from build123d import *

# Parameters (mm, degrees)
F0_W     = 274.9042
F0_H     = 560.5272
F1_DEPTH = 19.05
F3_DEPTH = 25.4
F4_W     = 50.8
F4_H     = 19.05
F5_DEPTH = 19.05
F7_DEPTH = 19.05
F8_R     = 50.8


with BuildPart() as f1:
    # F0 (on Top) → F1 (new body)
    with BuildSketch(Plane.XY):
        with Locations((-33.675123, 17.433073)):
            Rectangle(F0_W, F0_H)
    extrude(amount=F1_DEPTH)

    # F2 (on face) → F3 (cut)
    with BuildSketch(Plane.XY.offset(19.05)):
        Polygon((49.734686, 173.754715), (71.204288, 219.794873), (53.93326, 227.848758), (32.463658, 181.808599), align=None)
        Polygon((-21.578634, 65.918441), (-4.307605, 57.864557), (17.161997, 103.904715), (-0.109031, 111.958599), align=None)
        Polygon((-75.620925, -49.971717), (-58.349897, -58.025601), (-36.880294, -11.985443), (-54.151322, -3.931559), align=None)
        Polygon((-129.663216, -165.861875), (-112.392188, -173.915759), (-90.922585, -127.875601), (-108.193613, -119.821717), align=None)
    extrude(amount=-F3_DEPTH, mode=Mode.SUBTRACT)

    # F4 (on face) → F5 (join)
    with BuildSketch(Plane.XZ.offset(262.830527)):
        with Locations((-97.797423, 9.525)):
            Rectangle(F4_W, F4_H)
        with Locations((29.202577, 9.525)):
            Rectangle(F4_W, F4_H)
    extrude(amount=F5_DEPTH)

    # F6 (on face) → F7 (cut)
    with BuildSketch(Plane.XY.offset(19.05)):
        Polygon((-133.570358, -71.706755), (26.208879, 232.032016), (-133.570358, 232.032016), align=None)
    extrude(amount=-F7_DEPTH, mode=Mode.SUBTRACT)

    # F8
    f8_edges = [f1.edges().sort_by_distance(p)[0] for p in [
        (-171.127223, 297.696673, 9.525),
        (103.776977, 297.696673, 9.525),
    ]]
    fillet(f8_edges, radius=F8_R)


solid = f1.part
Model file for the job. Use its own axes, mm. A direction names the side the tool comes from. Round coordinates to 2 decimals unless told otherwise and drop trailing zeros. Loops run counter-clockwise (first coordinate to the right, second up) from the corner with the lowest first, then second, coordinate; pieces in that order, holes last.
1. Drop flat-ended pins along their axis: P1, Ø5.5, axis at y = -267.5, z = 6, coming from the -X side; P2, Ø5.5, axis at x = 75, z = 14, coming from the -Y side; P3, Ø5.5, axis at y = -267.5, z = 12, coming from the +X side. Give the stop position or say it passes through.
Check values:
P1: stops at x = -123.2
P2: stops at y = -262.83
P3: stops at x = 54.6
2. Wall check: probe 1 along Y at (x, z) = (-43, 2); probe 2 along Y at (x, z) = (-91, 9.75); probe 3 along X at (y, z) = (-6, 14.5). Give the ranges that are in metal, low to high.
Check values:
probe 1: y = -262.83 to -25.11, -9.13 to 100.47, 232.03 to 297.7
probe 2: y = -281.88 to -128.04, -127.84 to 9.22, 232.03 to 297.7
probe 3: x = -171.13 to -133.57, -99.01 to -55.12, -49.72 to 103.78
3. Mould opens along Y. For faces 1 (the flat face through (-171.127, -12, 9)), 2 (the flat face through (-119, -143, 10)), 3 (the cylindrical face through (-156.64, 282.42, 9.66)) say: +Y half, -Y half, draft (parallel to the pull), parting line (faces both ways), or undercut.
Check values:
face 1: draft
face 2: undercut
face 3: +Y half
4. Tool access for faces 4 (the flat face through (-64.736, -26.629, 9.658)), 5 (the flat face through (54.603, -272, 9)), 6 (the flat face through (-72.397, -272, 9)): list every direction of +Z, -Z, +X, -X, +Y, -Y with a clear straight run to the whole face (end or side of a thin tool).
Check values:
face 4: +Z, -Z
face 5: +Z, -Z, +X, -Y
face 6: +Z, -Z, -Y
5. Band-saw the part on A-A, the plane x = -66.5. List the corners of the cut face in (y, z), and give its area (3 significant figures).
Check values:
outline: (-262.83, 0) - (-54.23, 0) - (-54.23, 19.05) - (-262.83, 19.05) - close; (-30.41, 0) - (55.79, 0) - (55.79, 19.05) - (-30.41, 19.05) - close; (232.03, 0) - (297.7, 0) - (297.7, 19.05) - (232.03, 19.05) - close
area: 6,870 mm2
6. Band-saw the part on D-D, the plane y = 212. List the corners of the cut face in (x, z).
Check values:
outline: (-171.13, 0) - (-133.57, 0) - (-133.57, 19.05) - (-171.13, 19.05) - close; (15.67, 0) - (46.54, 0) - (46.54, 19.05) - (15.67, 19.05) - close; (67.57, 0) - (103.78, 0) - (103.78, 19.05) - (67.57, 19.05) - close
7. Band-saw the part on B-B, the plane z = 8. Count the separate pieces of the cut face and the enclosed holes in it, and give its area (3 significant figures).
Check values:
separate pieces: 1
enclosed holes: 5
area: 127,000 mm2
8. Band-saw the part on C-C, the plane y = 43.5. List the corners of the cut face in (x, z), and give its area (3 significant figures).
Check values:
outline: (-171.13, 0) - (-133.57, 0) - (-133.57, 19.05) - (-171.13, 19.05) - close; (-72.97, 0) - (103.78, 0) - (103.78, 19.05) - (-72.97, 19.05) - close
area: 4,080 mm2
